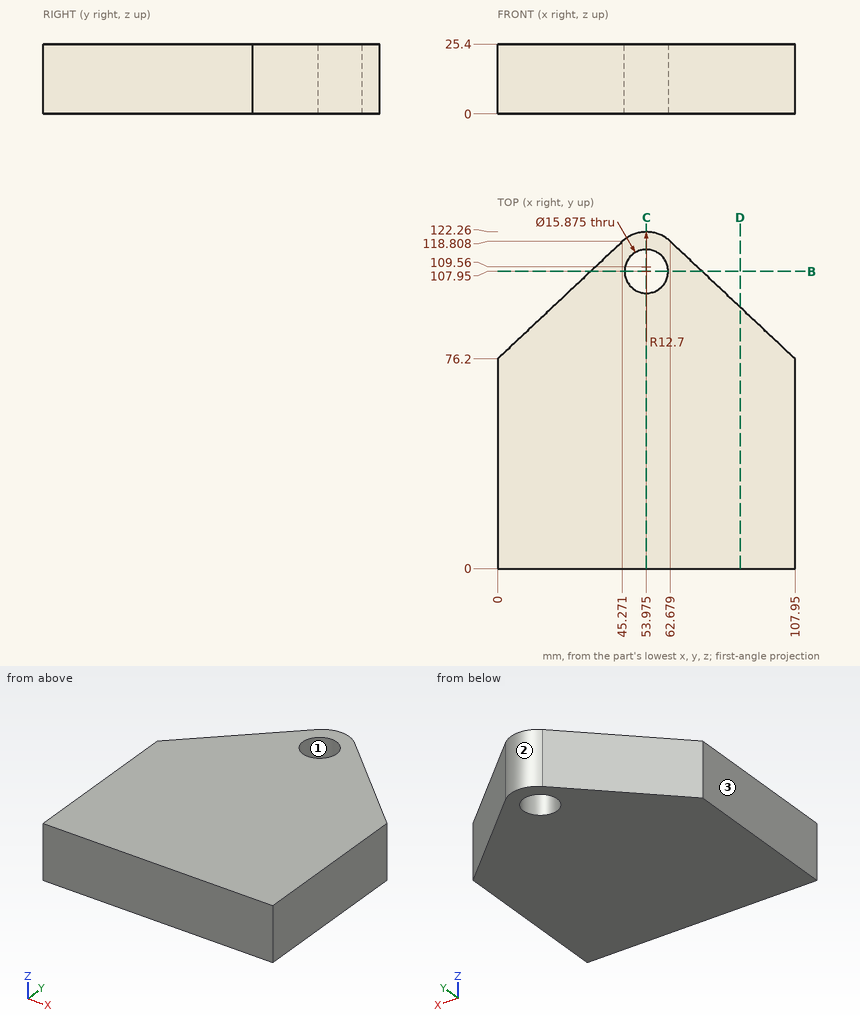
Part print with two shaded views. Sizes in mm from the minimum x, y, z corner. Round coordinates to 2 decimals unless told otherwise and drop trailing zeros. Order: outer loops, then holes, each group sorted by start corner. A loop starts at its lowest first (then second) coordinate and runs counter-clockwise, first axis right, second up. Notation, with made-up numbers: M -26,57.25 L 17,57.25 A12 cw 17,62.25 Z; hole C 7,24.25 d5. An arc over 180 degrees is marked long. Put each result on its own line as item: value. Start each with the question number.
1. Slice it at D-D on x = 88. List the corners of the cut face in (y, z), then the cut area to 3 significant figures.
2. Two-plate mould, pull along Y, no slides. Class the marked faces 1, 2 and 3: +Y half, -Y half, draft (parallel to the pull), parting line (faces both ways), or undercut.
3. Slice it at B-B on y = 107.95. List the corners of the cut face in (x, z), then the cut area to 3 significant figures.
4. Drop flat-ended pins along their axis: pin 1 (6 mm diameter, centred on x = 55.5, z = 21, fed in from -Y); pin 2 (5 mm diameter, centred on x = 90, z = 14.5, fed in from +Y); pin 3 (6 mm diameter, centred on y = 80, z = 15, fed in from -X); pin 4 (1 mm diameter, centred on x = 71.5, z = 20, fed in from +Y). Give the stop position or say it passes through.
5. Drill centre lines: probe 1 along Y at (x, z) = (20.5, 23) (1 decimal); probe 2 along Y at (x, z) = (23, 24.5); probe 3 along X at (y, z) = (82, 4.75). Where is each one in solid material? Low to high. Write a range as [from, to].
6. Slice it at C-C on x = 54. List the corners of the cut face in (y, z).
Findings:
1. outline: M 0,0 L 94.98,0 L 94.98,25.4 L 0,25.4 Z
1. area: 2,410 mm2
2. face 1: undercut
2. face 2: +Y half
2. face 3: draft
3. outline: M 33.73,0 L 46.04,0 L 46.04,25.4 L 33.73,25.4 Z; M 61.91,0 L 74.22,0 L 74.22,25.4 L 61.91,25.4 Z
3. area: 625 mm2
4. pin 1: y = 0
4. pin 2: y = 95.45
4. pin 3: x = 0.85
4. pin 4: y = 110.98
5. probe 1: [0, 95.5]
5. probe 2: [0, 97.85]
5. probe 3: [6.16, 101.79]
6. outline: M 0,0 L 100.01,0 L 100.01,25.4 L 0,25.4 Z; M 115.89,0 L 122.26,0 L 122.26,25.4 L 115.89,25.4 Z
